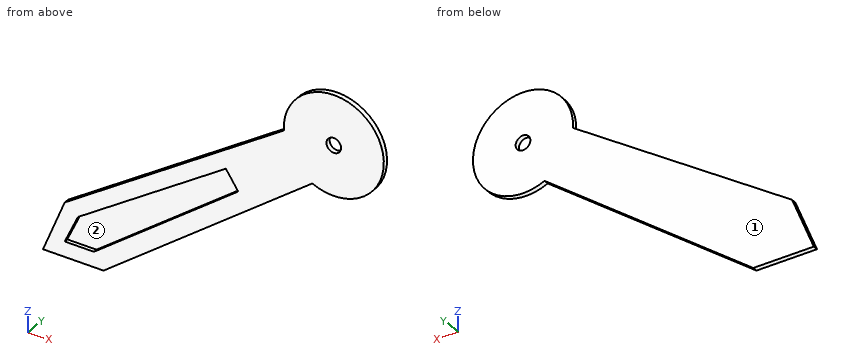
```python
from build123d import *

# Parameters (mm, degrees)
SKETCH1_R           = 0.15
BOSS_EXTRUDE1_DEPTH = 0.1
BOSS_EXTRUDE3_DEPTH = 0.02


with BuildPart() as part:
    # Sketch1 → Boss-Extrude1 (new body)
    with BuildSketch(Plane(origin=(0, 0, 0), x_dir=(1, 0, 0), z_dir=(0, 1, 0))):
        with BuildLine():
            Line((-5.928976917, 4.17249718), (-5.486197441, 3.071413653))
            Line((-5.486197441, 3.071413653), (-1.019009626, 0.054984583))
            ThreePointArc((-1.019009626, 0.054984583), (0.847824795, -0.567976267), (-0.438539423, 0.921459222))
            Line((-0.438539423, 0.921459222), (-4.694959938, 4.17249718))
            Line((-4.694959938, 4.17249718), (-5.928976917, 4.17249718))
        make_face()
        with Locations(Location((0, 0, 0), (0, 0, 270))):
            Circle(SKETCH1_R, mode=Mode.SUBTRACT)
        Polygon((-5.486197441, 3.860892642), (-5.216856249, 3.271495682), (-2.200234898, 1.239893548), (-1.948613115, 1.613513771), (-4.890993257, 3.860892642), align=None, mode=Mode.SUBTRACT)
    extrude(amount=BOSS_EXTRUDE1_DEPTH)

    # Sketch3 → Boss-Extrude3 (add)
    with BuildSketch(Plane(origin=(0, 0.1, 0), x_dir=(1, 0, 0), z_dir=(0, 1, 0))):
        Polygon((-5.669795802, 4.060835761), (-4.60725372, 3.952218978), (-1.551568417, 1.529417339), (-2.04496188, 0.980620035), (-5.388394983, 3.169960387), align=None)
    extrude(amount=-BOSS_EXTRUDE3_DEPTH)


solid = part.part
```
For this review, take the finished solid that the model builds, in its own axes (mm). Face numbers are marked on the shaded views. Coordinates: 2 decimals unless noted, no trailing zeros. Write each loop counter-clockwise with the first axis right and the second up, starting at its lowest first coordinate (ties: lowest second). Pieces come first, ordered by that corner, then holes.
(1) Add section A-A on x = 0. Give the boundary of the cut face in (y, z), then the cut area to 3 significant figures.
(2) Add section B-B on z = -2.7. Give the boundary of the cut face in (x, y), then the cut area to 3 significant figures.
(3) Add section D-D on z = -0.75. Give the boundary of the cut face in (x, y).
(4) For pin 1 Ø2 at (x, z) = (-5, -1) entering from +Y, flat-tipped, find the tip position at first contact; note if it passes through.
(5) The part is to be moulded in two halves that separate along Z. For the marked faces 1 and 2, say which applies: +Z half, -Z half, draft (parallel to the pull), parting line (faces both ways), or undercut.
(6) Wall thickness on probe 1 along X at (y, z) = (0.05, 0); probe 2 along Z at (x, y) = (0.75, 0.05): over which ranges is each line inside the solid? List them lowest first.
(7) Add section C-C on x = -3. Give the boundary of the cut face in (y, z), then the cut area to 3 significant figures.
Answer sheet:
1. outline: (0, -1.02) - (0.1, -1.02) - (0.1, -0.15) - (0, -0.15) - close; (0, 0.15) - (0.1, 0.15) - (0.1, 1.02) - (0, 1.02) - close
1. area: 0.174 mm2
2. outline: (-4.94, 0) - (-4.37, 0) - (-4.37, 0.08) - (-3.37, 0.08) - (-3.37, 0) - (-2.77, 0) - (-2.77, 0.1) - (-4.94, 0.1) - close
2. area: 0.137 mm2
3. outline: (-2.05, 0) - (0.69, 0) - (0.69, 0.1) - (-2.05, 0.1) - close
4. pin 1: passes through
5. face 1: draft
5. face 2: undercut
6. probe 1: x = -1.02 to -0.15, 0.15 to 1.02
6. probe 2: z = -0.69 to 0.69
7. outline: (0, -2.88) - (0.1, -2.88) - (0.1, -1.39) - (0, -1.39) - (0, -1.78) - (0.08, -1.78) - (0.08, -2.42) - (0, -2.42) - close
7. area: 0.0975 mm2
